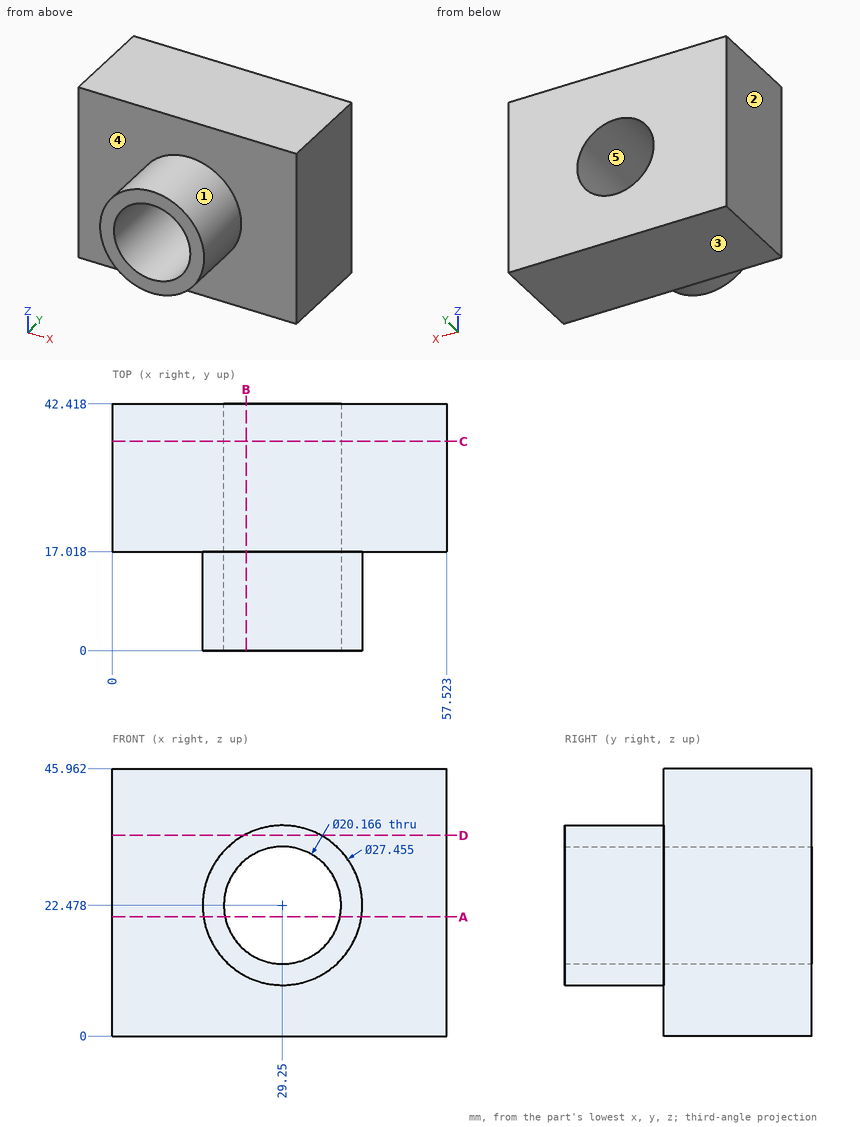
Source: three-view drawing plus pictorial views. Frame: mm from the lowest corner of the part. A direction names the side the tool comes from. Round coordinates to 2 decimals unless told otherwise and drop trailing zeros. Write each loop counter-clockwise with the first axis right and the second up, starting at its lowest first coordinate (ties: lowest second). Pieces come first, ordered by that corner, then holes. Notation, with made-up numbers: (28, 3.25) -> (60, 3.25) arc R17 cw to (60, 12.25) -> close; hole circle Ø3 at (65, -11.5). An arc over 180 degrees is marked (long way). Return JSON: item names as keys, results as strings.
Q1. Section B-B on x = 23. Return the cut outline in (y, z) (1 decimal).
From the geometry:
{"outline": "(0, 10.3) -> (17, 10.3) -> (17, 0) -> (42.4, 0) -> (42.4, 14.6) -> (0, 14.6) -> close; (0, 30.4) -> (42.4, 30.4) -> (42.4, 46) -> (17, 46) -> (17, 34.7) -> (0, 34.7) -> close"}
Q2. Set-up query: the marked faces 1 and 2. Return all of +Z, -Z, +X, -X, +Y, -Y with unobstructed straight access to the full face (end or side cutting, diameter ignored); none if empty.
From the geometry:
{"face 1": "-Y", "face 2": "+Z, -Z, -X, +Y, -Y"}
Q3. Ray query, line 1 (X direction, y = 17.5, z = 22); line 2 (Y direction, x = 23, z = 37); line 3 (X direction, y = 32, z = 15) (1 decimal). Return the intervals inside material, ascending.
From the geometry:
{"line 1": "0 to 19.18, 39.32 to 57.52", "line 2": "17.02 to 42.42", "line 3": "0 to 22.5, 36 to 57.5"}
Q4. Section D-D on z = 34.5. Return the cut outline in (x, y).
From the geometry:
{"outline": "(0, 17.02) -> (22.62, 17.02) -> (22.62, 0) -> (35.88, 0) -> (35.88, 17.02) -> (57.52, 17.02) -> (57.52, 42.42) -> (0, 42.42) -> close"}
Q5. First-contact query: pin 1 Ø4 at (y, z) = (10.5, 10.5) entering from -X; pin 2 Ø5 at (x, y) = (31.5, 9) entering from +Z (1 decimal); pin 3 Ø12 at (x, y) = (20.5, 5.5) entering from +Z; pin 4 Ø10 at (x, y) = (48.5, 10.5) entering from +Z. Flat tips, straight axial feed; report the tip coordinate or a pass-through.
From the geometry:
{"pin 1": "x = 19.82", "pin 2": "z = 36.2", "pin 3": "z = 35.93", "pin 4": "through"}
Q6. Mould query, pull axis Z, two halves, no side actions, for the marked faces 3, 4 and 5. Classes: +Z half, -Z half, draft (parallel to the pull), parting line (faces both ways), or undercut.
From the geometry:
{"face 3": "-Z half", "face 4": "draft", "face 5": "undercut"}
Q7. Section C-C on y = 36. Return the cut outline in (x, z).
From the geometry:
{"outline": "(0, 0) -> (57.52, 0) -> (57.52, 45.96) -> (0, 45.96) -> close; hole circle Ø20.17 at (29.25, 22.48)"}
Q8. Section A-A on z = 20.5. Return the cut outline in (x, y) (1 decimal).
From the geometry:
{"outline": "(0, 17) -> (15.7, 17) -> (15.7, 0) -> (19.4, 0) -> (19.4, 42.4) -> (0, 42.4) -> close; (39.1, 0) -> (42.8, 0) -> (42.8, 17) -> (57.5, 17) -> (57.5, 42.4) -> (39.1, 42.4) -> close"}
